Autodesk Fusion 360 part; units mm, degrees
sketch "Sketch1" plane through (0, 0, 0) normal (0, 1, 0) x (1, 0, 0)
  line L0 (193.9, 118.363) -> (193.9, 201.7255) construction
  line L1 (183.9, 190.7255) -> (183.9, 16)
  line L2 (23, 201.7255) -> (23, 118.363) construction
  line L3 (23, 12) -> (193.9, 12) construction
  circle A0 centre (23, 12) radius 3
  circle A1 centre (238.9, 12) radius 3
  line L4 (193.9, 95.3625) -> (23, 95.3625) construction
  line L5 (399.8, 190.7255) -> (399.8, 16)
  circle A2 centre (238.9, 95.3625) radius 3
  circle A3 centre (23, 201.7255) radius 3
  line L6 (33, 16) -> (33, 190.7255)
  line L7 (0, 212.7255) -> (0, 106.363) construction
  circle A4 centre (23, 118.363) radius 3
  circle A5 centre (193.9, 201.7255) radius 3
  circle A6 centre (23, 95.3625) radius 3
  line L8 (0, 106.3625) -> (0, 0) construction
  circle A7 centre (193.9, 95.3625) radius 3
  line L9 (23, 118.363) -> (193.9, 118.363) construction
  line L10 (193.9, 12) -> (193.9, 95.3625) construction
  circle A8 centre (193.9, 118.363) radius 3
  circle A9 centre (193.9, 12) radius 3
  line L11 (183.9, 16) -> (33, 16)
  line L12 (215.9, 0) -> (215.9, 106.3625) construction
  circle A10 centre (409.8, 118.363) radius 3
  line L13 (238.9, 118.363) -> (409.8, 118.363) construction
  line L14 (23, 95.3625) -> (23, 12) construction
  line L15 (215.9, 0) -> (431.8, 0) construction
  line L16 (431.8, 0) -> (431.8, 106.3625) construction
  line L17 (0, 106.363) -> (215.9, 106.363) construction
  circle A11 centre (409.8, 201.7255) radius 3
  line L18 (215.9, 106.3625) -> (0, 106.3625) construction
  line L19 (409.8, 201.7255) -> (238.9, 201.7255) construction
  line L20 (409.8, 12) -> (409.8, 95.3625) construction
  line L21 (215.9, 212.7255) -> (0, 212.7255) construction
  line L22 (0, 0) -> (215.9, 0) construction
  line L23 (215.9, 106.3625) -> (215.9, 0) construction
  circle A12 centre (409.8, 12) radius 3
  line L24 (215.9, 106.363) -> (431.8, 106.363) construction
  line L25 (409.8, 118.363) -> (409.8, 201.7255) construction
  line L26 (215.9, 106.363) -> (215.9, 212.7255) construction
  line L27 (238.9, 95.3625) -> (238.9, 12) construction
  circle A13 centre (409.8, 95.3625) radius 3
  line L28 (238.9, 12) -> (409.8, 12) construction
  line L29 (248.9, 16) -> (248.9, 190.7255)
  line L30 (248.9, 190.7255) -> (399.8, 190.7255)
  line L31 (431.8, 106.363) -> (431.8, 212.7255) construction
  line L32 (399.8, 16) -> (248.9, 16)
  line L33 (431.8, 212.7255) -> (215.9, 212.7255) construction
  line L34 (409.8, 95.3625) -> (238.9, 95.3625) construction
  line L35 (193.9, 201.7255) -> (23, 201.7255) construction
  line L36 (431.8, 106.3625) -> (215.9, 106.3625) construction
  line L37 (33, 190.7255) -> (183.9, 190.7255)
  circle A14 centre (238.9, 118.363) radius 3
  circle A15 centre (238.9, 201.7255) radius 3
  line L38 (238.9, 201.7255) -> (238.9, 118.363) construction
  line L39 (215.9, 212.7255) -> (215.9, 106.363) construction
  line L40 (432.8, 122.8753) -> (432.8, 213.7255)
  line L41 (432.8, 213.7255) -> (215.9, 213.7255)
  line L42 (215.9, 213.7255) -> (-1, 213.7255)
  line L43 (-1, 213.7255) -> (-1, 97.8373)
  line L44 (-1, 97.8373) -> (-1, -1)
  line L45 (-1, -1) -> (215.9, -1)
  line L46 (215.9, -1) -> (432.8, -1)
  line L47 (432.8, -1) -> (432.8, 122.8753)
  point P0 (215.9, 106.363)
  point P1 (0, 106.363)
  point P2 (215.9, 0)
  dimension "d3" = 215.9
  dimension "d4" = 106.363
  dimension "d5" = 106.3625
  dimension "d6" = 215.9
  dimension "d7" = 23
  dimension "d8" = 11
  dimension "d9" = 12
  dimension "d10" = 22
  dimension "d11" = 6
  dimension "d12" = 6
  dimension "d13" = 6
  dimension "d14" = 6
  dimension "d15" = 10
  dimension "d16" = 11
  dimension "d17" = 4
  dimension "d18" = 10
  dimension "d19" = 10
  dimension "d20" = 11
  dimension "d21" = 10
  dimension "d22" = 4
  dimension "d23" = 1
  dimension "d24" = 1
extrude "Extrude1" add sketch "Sketch1" along normal blind 5.4
sketch "Sketch2" plane through (0, 5.4, 0) normal (0, 1, 0) x (-1, 0, 0)
  circle A0 centre (-409.8, -12) radius 3
  circle A1 centre (-23, -95.3625) radius 3
  circle A2 centre (-409.8, -201.7255) radius 3
  circle A3 centre (-409.8, -95.3625) radius 3
  circle A4 centre (-238.9, -118.363) radius 3
  circle A5 centre (-238.9, -201.7255) radius 3
  circle A6 centre (-23, -12) radius 3
  circle A7 centre (-193.9, -201.7255) radius 3
  circle A8 centre (-193.9, -95.3625) radius 3
  line L0 (-399.8, -190.7255) -> (-399.8, -16)
  line L1 (-399.8, -16) -> (-248.9, -16)
  line L2 (-248.9, -16) -> (-248.9, -190.7255)
  line L3 (-248.9, -190.7255) -> (-399.8, -190.7255)
  circle A9 centre (-23, -201.7255) radius 3
  line L4 (-33, -16) -> (-33, -190.7255)
  line L5 (-33, -190.7255) -> (-183.9, -190.7255)
  line L6 (-183.9, -190.7255) -> (-183.9, -16)
  line L7 (-183.9, -16) -> (-33, -16)
  circle A10 centre (-23, -118.363) radius 3
  circle A11 centre (-238.9, -12) radius 3
  circle A12 centre (-238.9, -95.3625) radius 3
  circle A13 centre (-193.9, -118.363) radius 3
  circle A14 centre (-409.8, -118.363) radius 3
  circle A15 centre (-193.9, -12) radius 3
  line L8 (-432.8, 1) -> (-432.8, -122.8753)
  line L9 (-432.8, -122.8753) -> (-432.8, -213.7255)
  line L10 (-432.8, -213.7255) -> (1, -213.7255)
  line L11 (1, -213.7255) -> (1, -97.8373)
  line L12 (1, -97.8373) -> (1, 1)
  line L13 (1, 1) -> (-432.8, 1)
  line L14 (-399.8, -22) -> (-432.8, -22)
  line L15 (-432.8, -22) -> (-432.8, -82)
  line L16 (-432.8, -82) -> (-399.8, -82)
  line L17 (-399.8, -82) -> (-399.8, -22)
  dimension "d27" = 60
  dimension "d65" = 6
  dimension "d66" = 60
extrude "Extrude2" cut sketch "Sketch2" against normal blind 20 contours L0 L8 L14 L15 L16 L17
sketch "Sketch3" plane through (0, 5.4, 0) normal (0, 1, 0) x (-1, 0, 0)
  circle A0 centre (-193.9, -12) radius 3
  circle A1 centre (-409.8, -118.363) radius 3
  circle A2 centre (-193.9, -118.363) radius 3
  circle A3 centre (-238.9, -95.3625) radius 3
  circle A4 centre (-238.9, -12) radius 3
  circle A5 centre (-23, -118.363) radius 3
  line L0 (-33, -16) -> (-33, -190.7255)
  line L1 (-33, -190.7255) -> (-183.9, -190.7255)
  line L2 (-183.9, -190.7255) -> (-183.9, -16)
  line L3 (-183.9, -16) -> (-33, -16)
  circle A6 centre (-23, -201.7255) radius 3
  line L4 (-432.8, -22) -> (-399.8, -22)
  line L5 (-248.9, -16) -> (-248.9, -190.7255)
  line L6 (-248.9, -190.7255) -> (-399.8, -190.7255)
  line L7 (-399.8, -22) -> (-399.8, -16)
  line L8 (-399.8, -82) -> (-432.8, -82)
  line L9 (-432.8, -82) -> (-432.8, -122.8753)
  line L10 (-432.8, -122.8753) -> (-432.8, -213.7255)
  line L11 (-432.8, -213.7255) -> (1, -213.7255)
  line L12 (1, -213.7255) -> (1, -97.8373)
  line L13 (1, -97.8373) -> (1, 1)
  line L14 (1, 1) -> (-432.8, 1)
  line L15 (-432.8, 1) -> (-432.8, -22)
  circle A7 centre (-193.9, -95.3625) radius 3
  circle A8 centre (-193.9, -201.7255) radius 3
  circle A9 centre (-23, -12) radius 3
  circle A10 centre (-238.9, -201.7255) radius 3
  circle A11 centre (-238.9, -118.363) radius 3
  circle A12 centre (-409.8, -95.3625) radius 3
  circle A13 centre (-409.8, -201.7255) radius 3
  circle A14 centre (-23, -95.3625) radius 3
  circle A15 centre (-409.8, -12) radius 3
  line L16 (1, -213.7255) -> (6.4, -213.7255)
  line L17 (6.4, -213.7255) -> (6.4, -193.7255)
  line L18 (6.4, -193.7255) -> (1, -193.7255)
  line L19 (1, -193.7255) -> (1, -213.7255)
  line L20 (1, 1) -> (6.4, 1)
  line L21 (6.4, 1) -> (6.4, -19)
  line L22 (6.4, -19) -> (1, -19)
  line L23 (1, -19) -> (1, 1)
  line L24 (1, 1) -> (-19, 1)
  line L25 (-19, 1) -> (-19, 6.4)
  line L26 (-19, 6.4) -> (1, 6.4)
  line L27 (1, 6.4) -> (1, 1)
  line L28 (1, -213.7255) -> (-19, -213.7255)
  line L29 (-19, -213.7255) -> (-19, -219.1255)
  line L30 (-19, -219.1255) -> (1, -219.1255)
  line L31 (1, -219.1255) -> (1, -213.7255)
  line L32 (-432.8, -213.7255) -> (-412.8, -213.7255)
  line L33 (-412.8, -213.7255) -> (-412.8, -219.1255)
  line L34 (-412.8, -219.1255) -> (-432.8, -219.1255)
  line L35 (-432.8, -219.1255) -> (-432.8, -213.7255)
  line L36 (-432.8, -213.7255) -> (-438.2, -213.7255)
  line L37 (-438.2, -213.7255) -> (-438.2, -193.7255)
  line L38 (-438.2, -193.7255) -> (-432.8, -193.7255)
  line L39 (-432.8, -193.7255) -> (-432.8, -213.7255)
  line L40 (-432.8, 1) -> (-438.2, 1)
  line L41 (-438.2, 1) -> (-438.2, -19)
  line L42 (-438.2, -19) -> (-432.8, -19)
  line L43 (-432.8, -19) -> (-432.8, 1)
  line L44 (-432.8, 1) -> (-412.8, 1)
  line L45 (-412.8, 1) -> (-412.8, 6.4)
  line L46 (-412.8, 6.4) -> (-432.8, 6.4)
  line L47 (-432.8, 6.4) -> (-432.8, 1)
  line L48 (-399.8, -16) -> (-248.9, -16)
  line L49 (-399.8, -190.7255) -> (-399.8, -82)
  dimension "d30" = 5.4
  dimension "d31" = 20
  dimension "d32" = 5.4
  dimension "d33" = 20
  dimension "d34" = 20
  dimension "d35" = 5.4
  dimension "d36" = 5.4
  dimension "d37" = 20
  dimension "d38" = 20
  dimension "d39" = 5.4
  dimension "d40" = 5.4
  dimension "d41" = 20
  dimension "d42" = 5.4
  dimension "d43" = 20
  dimension "d44" = 20
  dimension "d45" = 5.4
  dimension "d63" = 433.8
extrude "Extrude3" add sketch "Sketch3" against normal blind 5.4 contours A0 | A1 | A2 | A3 | A4 | A5 | A6 | L4 L5 L6 L7 L8 L9 L10 L11 L12 L13 L14 L15 L19 L23 L24 L28 L32 L39 L43 L44 L48 L49 | L15 L40 L41 L42 L43 | L14 L44 L45 L46 L47 | L14 L24 L25 L26 L27 | L13 L20 L21 L22 L23 | L12 L16 L17 L18 L19 | L10 L36 L37 L38 L39 | L11 L28 L29 L30 L31 | L11 L32 L33 L34 L35 | A7 | A8 | A9 | A10 | A11 | A12 | A13 | A14 | A15
extrude "Extrude5" cut sketch "Sketch1" along normal blind 30 contours A0 | A1 | A2 | A3 | A4 | A5 | A6 | A7 | A8 | A9 | A10 | A11 | A12 | A13 | A14 | A15
sketch "export" plane through (0, 5.4, 0) normal (0, 1, 0) x (-1, 0, 0)
  circle A0 centre (-23, -118.363) radius 3
  circle A1 centre (-409.8, -201.7255) radius 3
  circle A2 centre (-193.9, -12) radius 3
  circle A3 centre (-238.9, -118.363) radius 3
  circle A4 centre (-193.9, -118.363) radius 3
  circle A5 centre (-409.8, -12) radius 3
  circle A6 centre (-238.9, -201.7255) radius 3
  circle A7 centre (-23, -95.3625) radius 3
  circle A8 centre (-23, -201.7255) radius 3
  circle A9 centre (-409.8, -118.363) radius 3
  circle A10 centre (-238.9, -12) radius 3
  circle A11 centre (-238.9, -95.3625) radius 3
  circle A12 centre (-193.9, -95.3625) radius 3
  circle A13 centre (-409.8, -95.3625) radius 3
  circle A14 centre (-193.9, -201.7255) radius 3
  circle A15 centre (-23, -12) radius 3
  line L0 (-33, -16) -> (-33, -190.7255)
  line L1 (-33, -190.7255) -> (-183.9, -190.7255)
  line L2 (-183.9, -190.7255) -> (-183.9, -16)
  line L3 (-183.9, -16) -> (-33, -16)
  line L4 (-432.8, -22) -> (-399.8, -22)
  line L5 (-399.8, -22) -> (-399.8, -16)
  line L6 (-399.8, -16) -> (-248.9, -16)
  line L7 (-248.9, -16) -> (-248.9, -190.7255)
  line L8 (-248.9, -190.7255) -> (-399.8, -190.7255)
  line L9 (-399.8, -190.7255) -> (-399.8, -82)
  line L10 (-399.8, -82) -> (-432.8, -82)
  line L11 (-432.8, -82) -> (-432.8, -122.8753)
  line L12 (-432.8, -122.8753) -> (-432.8, -193.7255)
  line L13 (-432.8, -193.7255) -> (-438.2, -193.7255)
  line L14 (-438.2, -193.7255) -> (-438.2, -213.7255)
  line L15 (-438.2, -213.7255) -> (-432.8, -213.7255)
  line L16 (-432.8, -213.7255) -> (-432.8, -219.1255)
  line L17 (-432.8, -219.1255) -> (-412.8, -219.1255)
  line L18 (-412.8, -219.1255) -> (-412.8, -213.7255)
  line L19 (-412.8, -213.7255) -> (-19, -213.7255)
  line L20 (-19, -213.7255) -> (-19, -219.1255)
  line L21 (-19, -219.1255) -> (1, -219.1255)
  line L22 (1, -219.1255) -> (1, -213.7255)
  line L23 (1, -213.7255) -> (6.4, -213.7255)
  line L24 (6.4, -213.7255) -> (6.4, -193.7255)
  line L25 (6.4, -193.7255) -> (1, -193.7255)
  line L26 (1, -193.7255) -> (1, -97.8373)
  line L27 (1, -97.8373) -> (1, -19)
  line L28 (1, -19) -> (6.4, -19)
  line L29 (6.4, -19) -> (6.4, 1)
  line L30 (6.4, 1) -> (1, 1)
  line L31 (1, 1) -> (1, 6.4)
  line L32 (1, 6.4) -> (-19, 6.4)
  line L33 (-19, 6.4) -> (-19, 1)
  line L34 (-19, 1) -> (-412.8, 1)
  line L35 (-412.8, 1) -> (-412.8, 6.4)
  line L36 (-412.8, 6.4) -> (-432.8, 6.4)
  line L37 (-432.8, 6.4) -> (-432.8, 1)
  line L38 (-432.8, 1) -> (-438.2, 1)
  line L39 (-438.2, 1) -> (-438.2, -19)
  line L40 (-438.2, -19) -> (-432.8, -19)
  line L41 (-432.8, -19) -> (-432.8, -22)
equation "d17 = 11.00 mm - 7 mm"
equation "d22 = d17"
equation "d30 = d36"
equation "d31 = d33"
equation "d32 = d36"
equation "d34 = d33"
equation "d35 = d36"
equation "d37 = d33"
equation "d38 = d33"
equation "d39 = d36"
equation "d40 = d36"
equation "d41 = d33"
equation "d42 = d36"
equation "d43 = d33"
equation "d44 = d33"
equation "d45 = d42"
equation "d48 = d33"
equation "d50 = ( d63 - d48 ) / 2"
equation "d66 = d27"
Build history of the part. All positions in model axes, mm. Give positions to 0.01 mm unless a question says otherwise; leave off trailing zeros. Order: outer loops, then holes, each group sorted by start corner. A loop starts at its lowest first (then second) coordinate and runs counter-clockwise, first axis right, second up. Notation, with made-up numbers: M 88,39.25 L 107,39.25 A21 ccw 107,56.25 Z; hole C -26,26 d1. An arc over 180 degrees is marked long. Put each result on its own line as item: value.
Item 1: Wall check: probe 1 along X at (y, z) = (5.25, -190); probe 2 along Z at (x, y) = (238.9, 3.15); probe 3 along Z at (x, y) = (24.5, 2.95). Give the ranges that are in metal, low to high.
Results are:
probe 1: -1 to 33, 183.9 to 248.9, 399.8 to 432.8
probe 2: -213.73 to -204.73, -198.73 to -121.36, -115.36 to -98.36, -92.36 to -15, -9 to 1
probe 3: -213.73 to -204.32, -199.13 to -120.96, -115.76 to -97.96, -92.76 to -14.6, -9.4 to 1
Item 2: Cut at B-B on x = 283.5. Write the cut outline in (y, z), then the cut area to 3 significant figures.
Results are:
outline: M 0,-213.73 L 5.4,-213.73 L 5.4,-190.73 L 0,-190.73 Z; M 0,-16 L 5.4,-16 L 5.4,1 L 0,1 Z
area: 216 mm2
Item 3: Drop flat-ended pins along their axis: pin 1 Ø2 at (x, y) = (84.5, 1) entering from +Z; pin 2 Ø1.6 at (y, z) = (1.5, -120) entering from +X; pin 3 Ø5.5 at (x, z) = (238.9, -12) entering from +Y; pin 4 Ø2.5 at (y, z) = (1.5, -123.5) entering from -X. Give the stop position or say it passes through.
Results are:
pin 1: z = 1
pin 2: x = 432.8
pin 3: through
pin 4: x = -1
Item 4: Cut at C-C on z = -167. Write the cut outline in (x, y).
Results are:
outline: M -1,0 L 33,0 L 33,5.4 L -1,5.4 Z; M 183.9,0 L 248.9,0 L 248.9,5.4 L 183.9,5.4 Z; M 399.8,0 L 432.8,0 L 432.8,5.4 L 399.8,5.4 Z
Item 5: Cut at D-D on x = 216. Write the cut outline in (y, z).
Results are:
outline: M 0,-213.73 L 5.4,-213.73 L 5.4,1 L 0,1 Z
Item 6: Cut at A-A on z = -67. Write the cut outline in (x, y), then the cut area to 3 significant figures.
Results are:
outline: M -1,0 L 33,0 L 33,5.4 L -1,5.4 Z; M 183.9,0 L 248.9,0 L 248.9,5.4 L 183.9,5.4 Z
area: 535 mm2
